Check sheet for the drawn part. Datum: minimum x, y, z corner. Units: mm. Coordinates: 2 decimals unless noted, no trailing zeros. Order: outer loops, then holes, each group sorted by start corner. A loop starts at its lowest first (then second) coordinate and runs counter-clockwise, first axis right, second up.
1. Thickness scan on line 1 (X direction, y = 12, z = 25); line 2 (Z direction, x = 25.4, y = 29.5) (3 decimals); line 3 (X direction, y = 12, z = 31). Record the ranges inside material, lowest first.
2. Draft check along Z on the marked faces 1, 2 and 3. Enter one of: released by +Z, released by -Z, zero draft, split by the parting line, or undercut.
3. Cross-section at C-C (x = 67). Enter the section's corners in (y, z).
4. Gauge pin test, flat ends, axial feed: pin 1 Ø8 at (x, z) = (67, 51.5) entering from +Y; pin 2 Ø5 at (y, z) = (10, 31.5) entering from +X; pin 3 Ø1 at (x, y) = (61.5, 11.5) entering from +Z; pin 4 Ø12 at (x, y) = (66.5, 13) entering from +Z. Record the tip position at first contact, or that the pin passes through.
5. Cross-section at D-D (z = 44). Enter the section's corners in (x, y), then the cut area to 3 significant figures.
6. Cross-section at A-A (y = 33.5). Enter the section's corners in (x, z) (3 decimals), then the cut area to 3 significant figures.
7. Cross-section at B-B (z = 24). Enter the section's corners in (x, y), then the cut area to 3 significant figures.
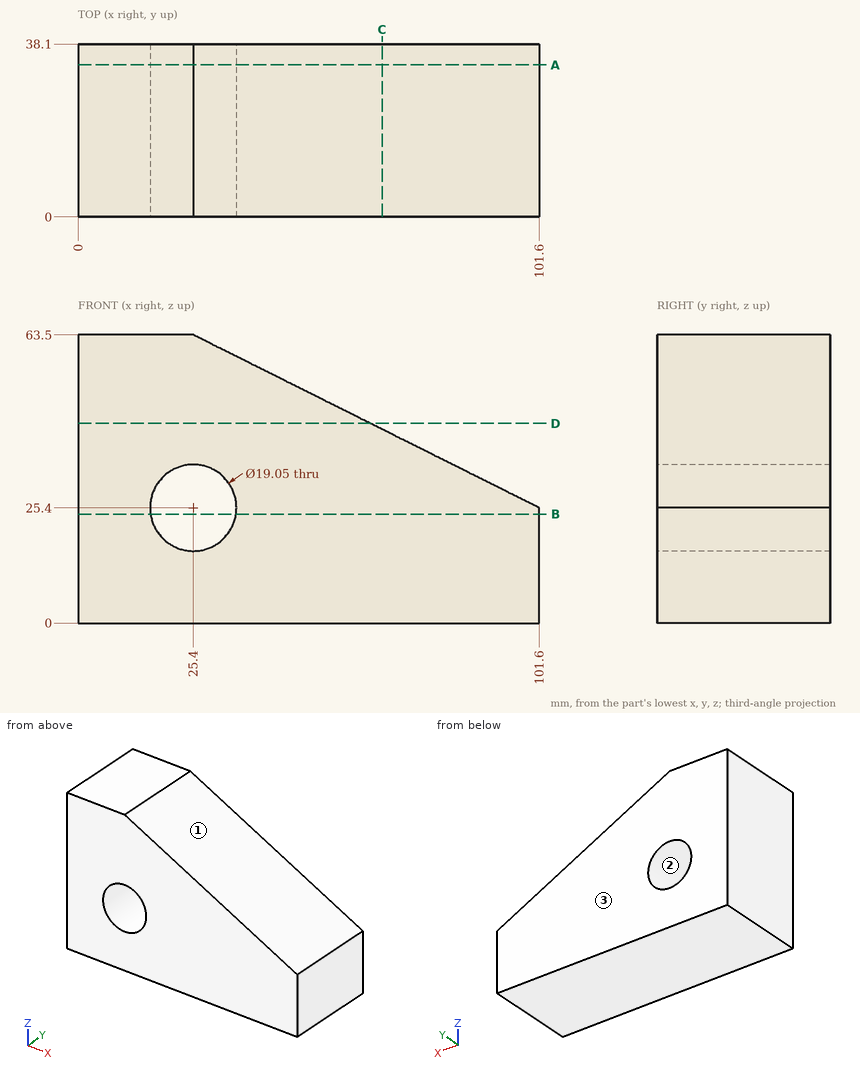
Data:
1. line 1: x = 0 to 15.88, 34.92 to 101.6
1. line 2: z = 0 to 15.875, 34.925 to 63.5
1. line 3: x = 0 to 17.7, 33.1 to 90.4
2. face 1: released by +Z
2. face 2: undercut
2. face 3: zero draft
3. outline: (0, 0) - (38.1, 0) - (38.1, 42.7) - (0, 42.7) - close
4. pin 1: passes through
4. pin 2: stops at x = 94.4
4. pin 3: stops at z = 45.7
4. pin 4: stops at z = 45.95
5. outline: (0, 0) - (64.4, 0) - (64.4, 38.1) - (0, 38.1) - close
5. area: 2,450 mm2
6. outline: (0, 0) - (101.6, 0) - (101.6, 25.4) - (25.4, 63.5) - (0, 63.5) - close; hole circle Ø19.05 at (25.4, 25.4)
6. area: 4,710 mm2
7. outline: (0, 0) - (15.98, 0) - (15.98, 38.1) - (0, 38.1) - close; (34.82, 0) - (101.6, 0) - (101.6, 38.1) - (34.82, 38.1) - close
7. area: 3,150 mm2
